Job drawing, mm, ordinate dimensions from the low corner. One solid piece. Give positions to 0.01 mm unless a question says otherwise; leave off trailing zeros. Order: outer loops, then holes, each group sorted by start corner. A loop starts at its lowest first (then second) coordinate and runs counter-clockwise, first axis right, second up.
Item 1: Band-saw the part on B-B on z = 6. Give the cut face in (x, y).
Item 2: Wall check: L1, parallel to Z at x = 6, y = 2.3; L2, parallel to X at y = 0.25, z = 5; L3, parallel to Z at x = 22.75, y = 3.65. Give the ranges that are in metal, low to high.
Item 3: Two-plate mould, pull along Z, no slides. Class the marked faces 1, 2, 3 and 4: released by +Z, released by -Z, zero draft, split by the parting line, or undercut.
Item 4: Flat gauge pins, fed straight in: P1, Ø2, axis at x = 22, z = 6, coming from the +Y side; P2, Ø5, axis at x = 6, z = 7.5, coming from the -Y side. Where does each tip first touch, or does it go through?
Item 5: Band-saw the part on C-C on y = 0.9. Give the cut face in (x, z), plus the area to 3 significant figures.
Item 6: Band-saw the part on D-D on x = 21.5. Give the cut face in (y, z), plus the area to 3 significant figures.
Item 7: Band-saw the part on A-A on x = 6. Give the cut face in (y, z), plus the area to 3 significant figures.
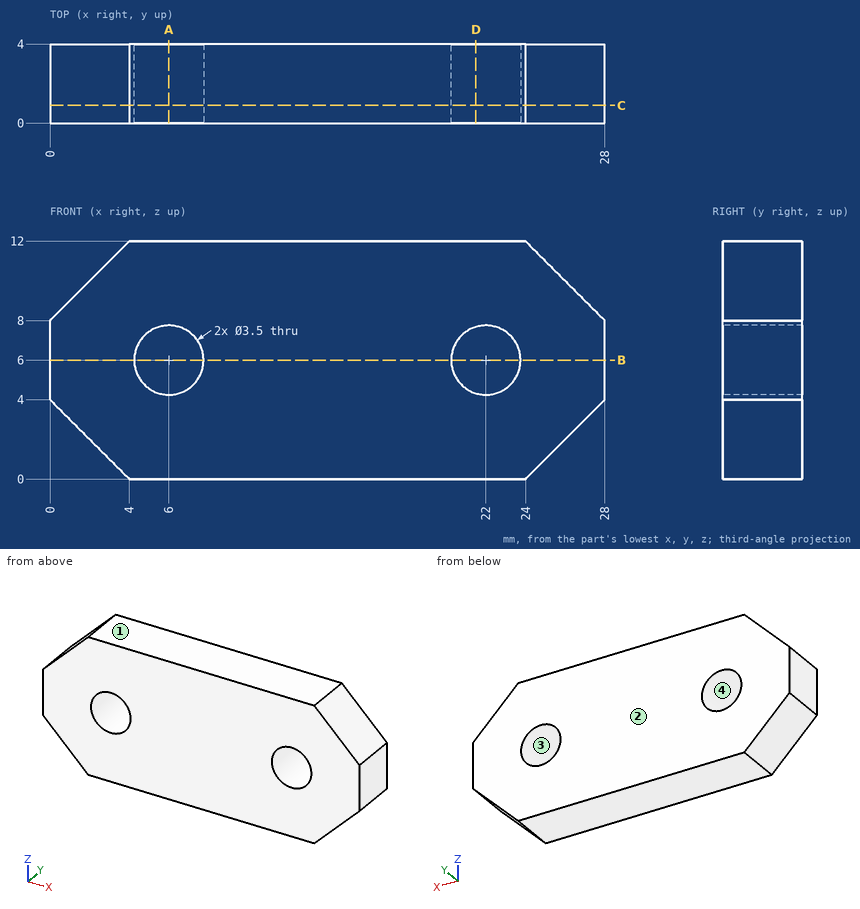
The answers:
1. outline: (0, 0) - (4.25, 0) - (4.25, 4) - (0, 4) - close; (7.75, 0) - (20.25, 0) - (20.25, 4) - (7.75, 4) - close; (23.75, 0) - (28, 0) - (28, 4) - (23.75, 4) - close
2. L1: z = 0 to 4.25, 7.75 to 12
2. L2: x = 0 to 4.56, 7.44 to 20.56, 23.44 to 28
2. L3: z = 0 to 4.42, 7.58 to 12
3. face 1: released by +Z
3. face 2: zero draft
3. face 3: undercut
3. face 4: undercut
4. P1: passes through
4. P2: stops at y = 0
5. outline: (0, 4) - (4, 0) - (24, 0) - (28, 4) - (28, 8) - (24, 12) - (4, 12) - (0, 8) - close; hole circle Ø3.5 at (6, 6); hole circle Ø3.5 at (22, 6)
5. area: 285 mm2
6. outline: (0, 0) - (4, 0) - (4, 4.32) - (0, 4.32) - close; (0, 7.68) - (4, 7.68) - (4, 12) - (0, 12) - close
6. area: 34.6 mm2
7. outline: (0, 0) - (4, 0) - (4, 4.25) - (0, 4.25) - close; (0, 7.75) - (4, 7.75) - (4, 12) - (0, 12) - close
7. area: 34.0 mm2
